Answer from the drawing. Dimensions are ordinates in mm from the lowest x, y and z of the part. Give positions to 0.01 mm unless a question says otherwise; leave off trailing zeros. Write each loop counter-clockwise with the first axis right and the second up, starting at its lowest first coordinate (ties: lowest second). Pieces come first, ordered by that corner, then holes.
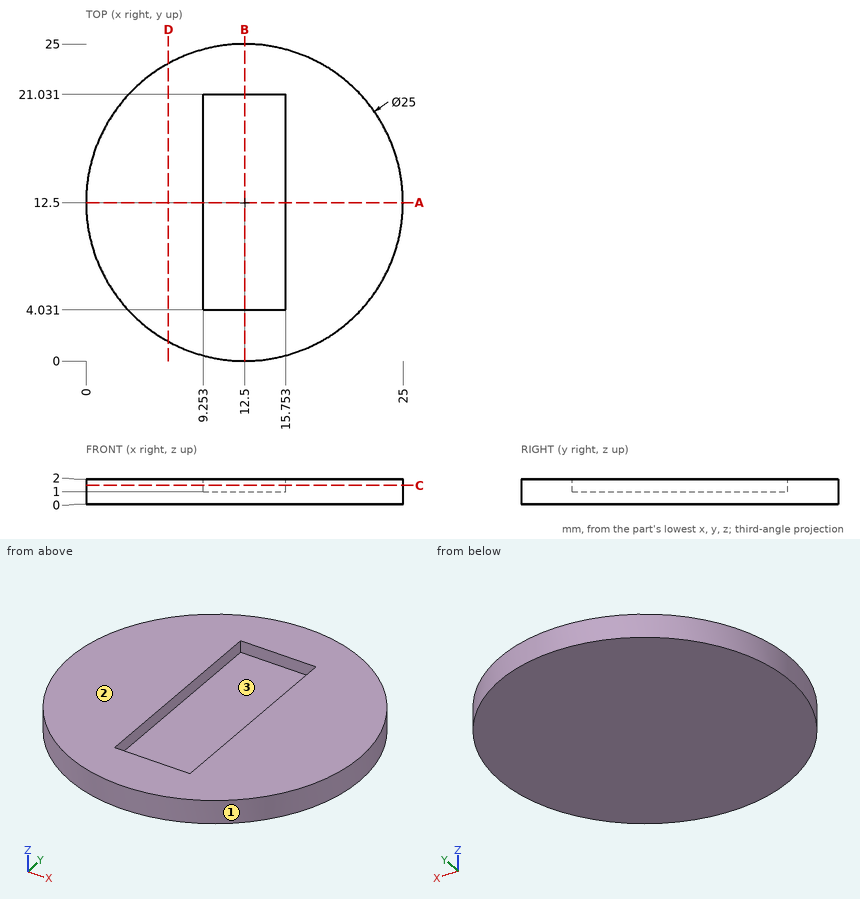
Item 1: Section D-D (x = 6.5) is taken. Write down the section's boundary in (y, z).
Result set:
outline: (1.53, 0) - (23.47, 0) - (23.47, 2) - (1.53, 2) - close
Item 2: Find the intervals of material crossed by line 1 along X through (y, z) = (16.25, 1.65) (1 decimal); line 2 along Y through (x, z) = (15, 1.65); line 3 along X through (y, z) = (12, 1.75), in increasing order.
Result set:
line 1: x = 0.6 to 9.3, 15.8 to 24.4
line 2: y = 0.25 to 4.03, 21.03 to 24.75
line 3: x = 0.01 to 9.25, 15.75 to 24.99
Item 3: Section B-B (x = 12.5) is taken. Write down the section's boundary in (y, z), and give its area (3 significant figures).
Result set:
outline: (0, 0) - (25, 0) - (25, 2) - (21.03, 2) - (21.03, 1) - (4.03, 1) - (4.03, 2) - (0, 2) - close
area: 33.0 mm2
Item 4: Section A-A (y = 12.5) is taken. Write down the section's boundary in (x, z), and give its area (3 significant figures).
Result set:
outline: (0, 0) - (25, 0) - (25, 2) - (15.75, 2) - (15.75, 1) - (9.25, 1) - (9.25, 2) - (0, 2) - close
area: 43.5 mm2
Item 5: Each of these flat-tipped pins is pushed along its axis until it touches: pin 1 Ø1 at (x, z) = (9, 1) entering from -Y (1 decimal); pin 2 Ø1.1 at (x, z) = (11.5, 1.5) entering from -Y; pin 3 Ø0.5 at (x, z) = (11.5, 1.5) entering from +Y. Where does it stop, or does it pass through?
Result set:
pin 1: stops at y = 0.4
pin 2: stops at y = 0.01
pin 3: stops at y = 24.98
Item 6: Section C-C (z = 1.5) is taken. Write down the section's boundary in (x, y).
Result set:
outline: circle Ø25 at (12.5, 12.5); hole (9.25, 4.03) - (15.75, 4.03) - (15.75, 21.03) - (9.25, 21.03) - close
Item 7: Determine the mould class of the marked faces 1, 2 and 3 for opening direction X: pulls with the +X half, pulls with the -X half, needs draft (parallel to the pull), parting line crosses it, or undercut.
Result set:
face 1: parting line crosses it
face 2: needs draft
face 3: undercut
